```python
from build123d import *

# Parameters (mm, degrees)
F1_DEPTH = 5.08
F2_W     = 8.89
F2_H     = 5.08
F3_DEPTH = 5.08


with BuildPart() as f1:
    # F0 (on Front) → F1 (new body)
    with BuildSketch(Plane.XZ):
        with BuildLine():
            Line((146.05, 0), (32.91078, 0))
            Line((32.91078, 0), (32.91078, -11.1125))
            ThreePointArc((32.91078, -11.1125), (43.013568, -15.297212), (47.19828, -25.4))
            ThreePointArc((47.19828, -25.4), (32.91078, -39.6875), (18.62328, -25.4))
            Line((18.62328, -25.4), (0, -25.4))
            Line((0, -25.4), (0, -139.7))
            Line((0, -139.7), (146.05, -139.7))
            Line((146.05, -139.7), (146.05, 0))
        make_face()
        with BuildLine():
            Line((32.91078, 0), (0, 0))
            Line((0, 0), (0, -25.4))
            Line((0, -25.4), (18.62328, -25.4))
            ThreePointArc((18.62328, -25.4), (22.807992, -15.297212), (32.91078, -11.1125))
            Line((32.91078, -11.1125), (32.91078, 0))
        make_face()
    extrude(amount=F1_DEPTH)

    # F2 (on face) → F3 (cut)
    with BuildSketch(Plane(origin=(0, 0, -139.7), x_dir=(1, 0, 0), z_dir=(0, 0, -1))):
        with Locations((4.445, 2.54)):
            Rectangle(F2_W, F2_H)
        with Locations((141.605, 2.54)):
            Rectangle(F2_W, F2_H)
    extrude(amount=-F3_DEPTH, mode=Mode.SUBTRACT)


solid = f1.part
```
Check sheet for the modelled part. Datum: model origin and axes. Units: mm. A direction names the side the tool comes from. Coordinates: 2 decimals unless noted, no trailing zeros. Order: outer loops, then holes, each group sorted by start corner. A loop starts at its lowest first (then second) coordinate and runs counter-clockwise, first axis right, second up. Notation, with made-up numbers: (-19, 3.25) -> (-11, 3.25) arc R11 ccw to (-11, 12.25) -> close; hole circle Ø2 at (58, 45.5). An arc over 180 degrees is marked (long way). Write item = value, one per line. Start each with the question number.
1) Access from +Z, -Z, +X, -X, +Y, -Y to the whole of each face (thin tool, end or side, straight path). Record for faces 1 (the flat face through (72, -3, -139.7)), 2 (the flat face through (137.16, -3, -137)), 3 (the flat face through (4, -3, -134.62)).
2) Cross-section at C-C (x = 41). Enter the section's corners in (y, z), then the cut area to 3 significant figures.
3) Go/stop test with flat-tipped pins: P1, Ø1.5, axis at y = -3, z = -137.5, coming from the +X side; P2, Ø1.5, axis at y = -3.5, z = -138.5, coming from the -X side. Record where each tip stops, or that it passes through.
4) Material ranges on L1, parallel to Z at x = 33.5, y = -0.95; L2, parallel to X at y = -1.85, z = -38; L3, parallel to X at y = -2.7, z = -36.5, recorded low to high.
5) Cross-section at B-B (x = 22). Enter the section's corners in (y, z), then the cut area to 3 significant figures.
Ans:
q1.face_1 = -Z, +X, -X, +Y, -Y
q1.face_2 = -Z, +X, +Y, -Y
q1.face_3 = -Z, -X, +Y, -Y
q2.outline = (-5.08, -139.7) -> (0, -139.7) -> (0, -37.18) -> (-5.08, -37.18) -> close; (-5.08, -13.62) -> (0, -13.62) -> (0, 0) -> (-5.08, 0) -> close
q2.area = 590 mm²
q3.P1 = 137.16
q3.P2 = 8.89
q4.L1 = -139.7 to -39.68, -11.12 to 0
q4.L2 = 0 to 26.17, 39.65 to 146.05
q4.L3 = 0 to 23.92, 41.91 to 146.05
q5.outline = (-5.08, -139.7) -> (0, -139.7) -> (0, -34.62) -> (-5.08, -34.62) -> close; (-5.08, -16.18) -> (0, -16.18) -> (0, 0) -> (-5.08, 0) -> close
q5.area = 616 mm²
